Read the model definition and answer for the solid it produces. Units are mm, in the model's axes. A direction names the side the tool comes from. Coordinates: 2 decimals unless noted, no trailing zeros. Order: outer loops, then holes, each group sorted by start corner. A loop starts at its lowest first (then second) coordinate and runs counter-clockwise, first axis right, second up.
from build123d import *

# Parameters (mm, degrees)
F1_DEPTH       = 2.5
F0_W           = 10.07359
F0_H           = 4
F0_W_2         = 10
F0_H_2         = 2
F2_DEPTH       = 20
F4_D           = 2
F4_CSINK_D     = 5
F4_CSINK_ANGLE = 90


with BuildPart() as f1:
    # F0 (on Top) → F1 (new body)
    with BuildSketch(Plane.XY):
        Polygon((9.374975, 18.726558), (-30.625025, 18.726558), (-30.625025, -6.273442), (9.374975, -6.273442), (9.374975, 16.726558), align=None)
        Polygon((-40.625025, 18.726558), (-30.625025, 18.726558), (9.374975, 18.726558), (9.374975, 20.726558), (19.374975, 20.726558), (19.374975, 28.726558), (-40.625025, 28.726558), (-40.625025, 27.726558), (-30.551435, 27.726558), (-30.551435, 23.726558), (-40.625025, 23.726558), align=None)
    extrude(amount=F1_DEPTH)

    # F0 (on Top) → F2 (join)
    with BuildSketch(Plane.XY):
        with Locations((-35.58823, 25.726558)):
            Rectangle(F0_W, F0_H)
        with Locations((14.374975, 19.726558)):
            Rectangle(F0_W_2, F0_H_2)
        with Locations((14.374975, 17.726558)):
            Rectangle(F0_W_2, F0_H_2)
    extrude(amount=F2_DEPTH)

    # F4 (through all)
    with Locations(Plane.XY.offset(2.5)):
        with Locations((-20.625025, -4.273442)):
            CounterSinkHole(F4_D / 2, F4_CSINK_D / 2, counter_sink_angle=F4_CSINK_ANGLE)


solid = f1.part
Q1. Determine the mould class of faces 1 (the cylindrical face through (-19.626, -4.229, 0.493)), 2 (the flat face through (14, 19, 20)), 3 (the flat face through (9.375, 5, 1)) for opening direction X: +X half, -X half, draft (parallel to the pull), parting line (faces both ways), or undercut.
Q2. Straight lines are drawn through the part: L1, parallel to X at y = 19, z = 5.25; L2, parallel to X at y = 26, z = 12; L3, parallel to Z at x = -21.5, y = -1. For each, find the intervals that lie inside material, in ascending order.
Q3. The part is cut by section B-B, the plane y = 25. Determine the outline of the cut face in (x, z).
Q4. Each of these flat-tipped pins is pushed along its axis until it touches: P1, Ø5, axis at x = 11.5, y = 13.5, coming from the +Z side; P2, Ø11, axis at x = -37, z = 11.5, coming from the +Y side; P3, Ø1.2, axis at y = 19, z = 10, coming from the -X side (3 decimals). Where does it stop, or does it pass through?
Q5. The part is cut by section D-D, the plane x = -13. Determine the outline of the cut face in (y, z).
Q6. The part is cut by section C-C, the plane x = 13.5. Determine the outline of the cut face in (y, z), then the cut area to 3 significant figures.
Q7. The part is cut by section A-A, the plane z = 10.5. Determine the outline of the cut face in (x, y), then the cut area to 3 significant figures.
Q8. Which of the six approach directions +Z, -Z, +X, -X, +Y, -Y give full straight-line access (tool end or side, diameter ignored) to faces 4 (the flat face through (14, 20.727, 11)), 5 (the flat face through (-36, 18.727, 1)), 6 (the flat face through (9.375, 19, 11))?
Computed values:
1. face 1: undercut
1. face 2: draft
1. face 3: +X half
2. L1: x = 9.37 to 19.37
2. L2: x = -40.63 to -30.55
2. L3: z = 0 to 2.5
3. outline: (-40.63, 0) - (19.37, 0) - (19.37, 2.5) - (-30.55, 2.5) - (-30.55, 20) - (-40.63, 20) - close
4. P1: stops at z = 2.5
4. P2: stops at y = 27.73
4. P3: stops at x = 9.375
5. outline: (-6.27, 0) - (28.73, 0) - (28.73, 2.5) - (-6.27, 2.5) - close
6. outline: (16.73, 0) - (28.73, 0) - (28.73, 2.5) - (20.73, 2.5) - (20.73, 20) - (16.73, 20) - close
6. area: 100 mm2
7. outline: (-40.63, 23.73) - (-30.55, 23.73) - (-30.55, 27.73) - (-40.63, 27.73) - close; (9.37, 16.73) - (19.37, 16.73) - (19.37, 20.73) - (9.37, 20.73) - close
7. area: 80.3 mm2
8. face 4: +Z, +X, -X, +Y
8. face 5: +Z, -Z, -X, -Y
8. face 6: +Z, -X, +Y, -Y
